Can you work these out from the model? Positions are in its coordinate system, mm. Face numbers are marked on the shaded views. A direction names the side the tool comes from. Give positions to 0.01 mm unless a question says otherwise; leave off trailing zeros. Write each loop counter-clockwise with the first axis right and the second up, starting at its lowest first coordinate (ties: lowest second). Pieces come first, ordered by that corner, then holes. Notation, with made-up numbers: (31.5, -9.75) - (58.5, -9.75) arc R35 cw to (58.5, 26.25) - close; hole circle Ø1 at (72.5, -21). An arc over 180 degrees is marked (long way). Return JSON: item names as keys, results as strings. Group by question number.
from build123d import *

# Parameters (mm, degrees)
SKETCH1_R           = 9.062508511
BOSS_EXTRUDE1_DEPTH = 3.5
CIRPATTERN1_COUNT   = 25
SKETCH3_R           = 4
BOSS_EXTRUDE2_DEPTH = 2
SKETCH2_R           = 1.25
CUT_EXTRUDE1_DEPTH  = 6.5


with BuildPart() as part:
    # Sketch1 → Boss-Extrude1 (new body)
    with BuildSketch(Plane.XY):
        with BuildLine():
            ThreePointArc((0, -29.062508511), (-0.402627944, -29.465136456), (-0.55, -30.015136456))
            Line((-0.55, -30.015136456), (-0.498437968, -30.951208914))
            ThreePointArc((-0.498437968, -30.951208914), (0, -30.937491489), (0.498437968, -30.951208914))
            Line((0.498437968, -30.951208914), (0.55, -30.015136456))
            ThreePointArc((0.55, -30.015136456), (0.402627944, -29.465136456), (0, -29.062508511))
        make_face()
        with Locations((0, -40)):
            Circle(SKETCH1_R)
    boss_extrude1 = extrude(amount=BOSS_EXTRUDE1_DEPTH)

    # CirPattern1: Boss-Extrude1 ×25 about axis
    cirpattern1_axis = Axis((0, -40, 0), (0, 0, 1))
    for i in range(1, CIRPATTERN1_COUNT):
        add(boss_extrude1.rotate(cirpattern1_axis, i * 360 / CIRPATTERN1_COUNT))

    # Sketch3 → Boss-Extrude2 (add)
    with BuildSketch(Plane(origin=(0, 0, 0), x_dir=(-1, 0, 0), z_dir=(0, 0, -1))):
        with Locations((0, -40)):
            Circle(SKETCH3_R)
    extrude(amount=BOSS_EXTRUDE2_DEPTH)

    # Sketch2 → Cut-Extrude1 (cut, through all)
    with BuildSketch(Plane.XY.offset(3.5)):
        with Locations((0, -40)):
            Circle(SKETCH2_R)
    extrude(amount=-CUT_EXTRUDE1_DEPTH, mode=Mode.SUBTRACT)


solid = part.part
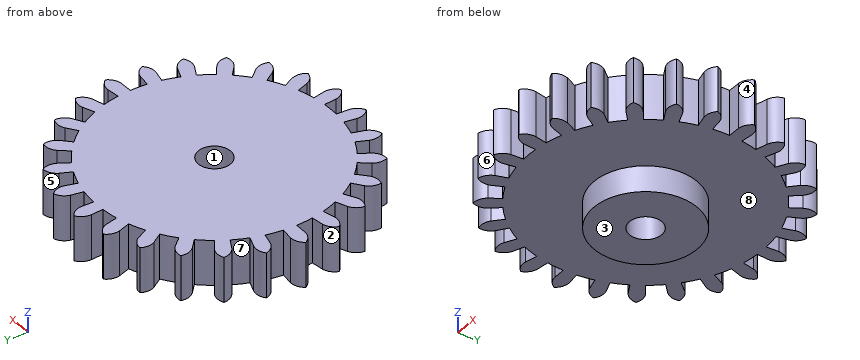
1) On a 3-axis mill with a long thin cutter (end or side, diameter ignored), from which of +Z, -Z, +X, -X, +Y, -Y can I reach the whole of each face in a straight line? I mean the marked faces 5, 6, 7 and 8. Say none if no direction works.
2) Imagine slicing it at A-A, the plane x = -2.25. Write out the boundary of the cut face in (y, z).
3) We'd pull the mould along X, two halves only. Please class the marked faces 1, 2, 3 and 4: pulls with the +X half, pulls with the -X half, needs draft (parallel to the pull), parting line crosses it, or undercut.
4) I need wall thicknesses on line 1 along X through (y, z) = (-30.75, 1.1); line 2 along Z through (x, y) = (0.75, -36); line 3 along Y through (x, z) = (-6, 0.95). Which ranges of each line are inside material? Lowest first, please.
5) Will these pins go through, and if not, where does the flat tip stop? pin 1 Ø5 at (x, y) = (-0.5, -39) entering from +Z; pin 2 Ø1 at (y, z) = (-46, 0) entering from -X; pin 3 Ø2 at (y, z) = (-34, 2) entering from +X.
Resolved:
{
 "1": {"face 5": "+Z, -Z, +Y", "face 6": "+Z, -Z, -Y", "face 7": "+Z, -Z", "face 8": "-Z"},
 "2": {"outline": "(-48.78, 0) - (-43.31, 0) - (-43.31, -2) - (-36.69, -2) - (-36.69, 0) - (-29.68, 0) - (-29.68, 3.5) - (-48.78, 3.5) - close"},
 "3": {"face 1": "undercut", "face 2": "pulls with the -X half", "face 3": "needs draft", "face 4": "pulls with the +X half"},
 "4": {"line 1": "-5.4 to -4.5, -2.93 to -1.84, -0.51 to 0.51, 1.84 to 2.93, 4.5 to 5.4", "line 2": "0 to 3.5", "line 3": "-48.81 to -47.37, -46.79 to -32.86"},
 "5": {"pin 1": "z = 3.5", "pin 2": "x = -8.4", "pin 3": "x = 9.24"}
}
